Design review of the part built by this model. Coordinates are the model's own, in mm. Coordinates: 2 decimals unless noted, no trailing zeros. Loops run counter-clockwise (first coordinate to the right, second up) from the corner with the lowest first, then second, coordinate; pieces in that order, holes last. Notation, with made-up numbers: M 85.25,11 L 136.25,11 A34 ccw 136.25,46 Z; hole C 29.5,21.5 d5. An arc over 180 degrees is marked long. Answer as a JSON object with one key per item and string values. Group by question number.
1. Consider section D-D (x = 13). State the section outline as (y, z) points.
2. Draft analysis for pull direction Y (two halves, no side actions). For faces 1 (the cylindrical face through (-0.35, 6.89, 4.82)), 2 (the cylindrical face through (-2.994, 22.804, 4.19)), 3 (the flat face through (-4, 23, 8.5)), state which applies: +Y half, -Y half, draft (parallel to the pull), parting line (faces both ways), or undercut.
3. To check wall thickness, follow probe 1 along Y at (x, z) = (0, 6); probe 2 along Y at (x, z) = (-7.5, 4.25); probe 3 along X at (y, z) = (8, 3). State the ranges of each line that lie inside material, in increasing order.
4. Consider section B-B (y = 0). State the section outline as (x, z) points.
5. Consider section A-A (x = 0). State the section outline as (y, z) points.
6. Insertion check: pin 1 (5 mm diameter, centred on x = -15.5, z = 3.5, fed in from -Y); pin 2 (1.5 mm diameter, centred on x = 13, z = 2, fed in from -Y); pin 3 (2 mm diameter, centred on y = 14.5, z = 5, fed in from +X). Each pin has a flat end and moves straight along its axis. Give the tip position at first contact, or say it passes through.
7. Consider section C-C (z = 7). State the section outline as (x, y) points (3 decimals).
from build123d import *

# Parameters (mm, degrees)
SKETCH1_R           = 23
SKETCH1_R_2         = 3.7
BOSS_EXTRUDE1_DEPTH = 9.5
BOSS_EXTRUDE3_START = -1
SKETCH9_R           = 25.5
SKETCH9_R_2         = 23
BOSS_EXTRUDE3_DEPTH = 1
HOLE1_D             = 3.2


with BuildPart() as part:
    # Sketch1 → Boss-Extrude1 (new body)
    with BuildSketch(Plane.XY):
        Circle(SKETCH1_R)
        Circle(SKETCH1_R_2, mode=Mode.SUBTRACT)
    extrude(amount=BOSS_EXTRUDE1_DEPTH)

    # Sketch9 → Boss-Extrude3 (add)
    with BuildSketch(Plane.XY.offset(9.5).offset(BOSS_EXTRUDE3_START)):
        Circle(SKETCH9_R)
        Circle(SKETCH9_R_2, mode=Mode.SUBTRACT)
    extrude(amount=BOSS_EXTRUDE3_DEPTH)

    # Hole1 (through all)
    with Locations(Plane(origin=(0, 8.45, 0), x_dir=(-1, 0, 0), z_dir=(0, 0, -1))):
        with Locations((0, 0), (-7.317914662, -12.675), (7.317914662, -12.675)):
            Hole(HOLE1_D / 2)


solid = part.part
Findings below:
{
 "1": {"outline": "M -21.94,8.5 L -18.97,8.5 L -18.97,0 L 18.97,0 L 18.97,8.5 L 21.94,8.5 L 21.94,9.5 L -21.94,9.5 Z"},
 "2": {"face 1": "undercut", "face 2": "parting line", "face 3": "draft"},
 "3": {"probe 1": "y = -23 to -3.7, 3.7 to 6.85, 10.05 to 23", "probe 2": "y = -21.74 to -5.81, -2.64 to 21.74", "probe 3": "x = -21.56 to -1.54, 1.54 to 21.56"},
 "4": {"outline": "M -25.5,8.5 L -23,8.5 L -23,0 L -3.7,0 L -3.7,9.5 L -25.5,9.5 Z; M 3.7,0 L 23,0 L 23,8.5 L 25.5,8.5 L 25.5,9.5 L 3.7,9.5 Z"},
 "5": {"outline": "M -25.5,8.5 L -23,8.5 L -23,0 L -3.7,0 L -3.7,9.5 L -25.5,9.5 Z; M 3.7,0 L 6.85,0 L 6.85,9.5 L 3.7,9.5 Z; M 10.05,0 L 23,0 L 23,8.5 L 25.5,8.5 L 25.5,9.5 L 10.05,9.5 Z"},
 "6": {"pin 1": "stops at y = -18.97", "pin 2": "stops at y = -19.47", "pin 3": "stops at x = 18.62"},
 "7": {"outline": "C 0,0 d46; hole C -7.318,-4.225 d3.2; hole C 0,0 d7.4; hole C 0,8.45 d3.2; hole C 7.318,-4.225 d3.2"}
}
